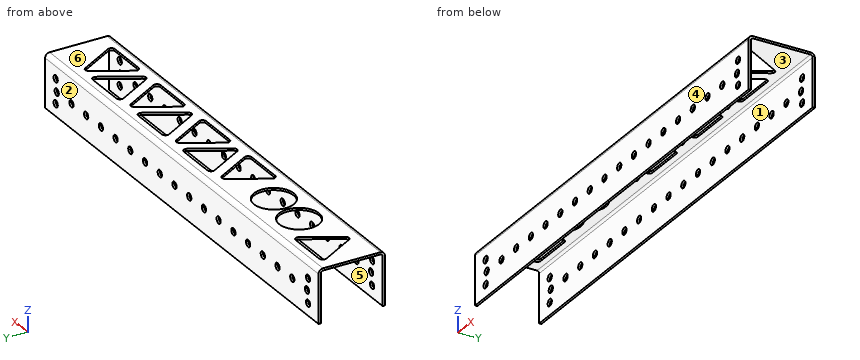
from build123d import *

# Parameters (mm, degrees)
BASE_FLANGE1_DEPTH = 165.1
SKETCH6_R          = 2.54
CUT_EXTRUDE1_DEPTH = 173.973769801
SKETCH8_R          = 14.2875
CUT_EXTRUDE2_DEPTH = 172.104223081
SKETCH9_R          = 14.2875
CUT_EXTRUDE3_DEPTH = 2.54
CUT_EXTRUDE4_DEPTH = 2.54
SKETCH11_R         = 2.54
CUT_EXTRUDE5_DEPTH = 173.973769801


# Sheet-metal steps are written as plain solids
with BuildPart() as part:
    # Sketch1 → Base-Flange1 (new, symmetric)
    with BuildSketch(Plane(origin=(0, 0, 0), x_dir=(0, 0, -1), z_dir=(1, 0, 0))):
        with BuildLine():
            Line((18.25625, 22.225), (-16.66875, 22.225))
            ThreePointArc((-16.66875, 22.225), (-17.791282015, 21.760032015), (-18.25625, 20.6375))
            Line((-18.25625, 20.6375), (-18.25625, -20.6375))
            ThreePointArc((-18.25625, -20.6375), (-17.791282015, -21.760032015), (-16.66875, -22.225))
            Line((-16.66875, -22.225), (18.25625, -22.225))
            Line((18.25625, -22.225), (18.25625, -23.8125))
            Line((18.25625, -23.8125), (-16.66875, -23.8125))
            ThreePointArc((-16.66875, -23.8125), (-18.91381403, -22.88256403), (-19.84375, -20.6375))
            Line((-19.84375, -20.6375), (-19.84375, 20.6375))
            ThreePointArc((-19.84375, 20.6375), (-18.91381403, 22.88256403), (-16.66875, 23.8125))
            Line((-16.66875, 23.8125), (18.25625, 23.8125))
            Line((18.25625, 23.8125), (18.25625, 22.225))
        make_face()
    extrude(amount=BASE_FLANGE1_DEPTH, both=True)

    # Sketch6 → Cut-Extrude1 (cut, through all)
    with BuildSketch(Plane(origin=(0, 23.8125, 0), x_dir=(1, 0, 0), z_dir=(0, 1, 0))):
        with Locations(Location((151.13, 0.79375, 0), (0, 0, 270))):
            Circle(SKETCH6_R)
        with Locations(Location((133.35, 0.79375, 0), (0, 0, 270))):
            Circle(SKETCH6_R)
        with Locations(Location((115.57, 0.79375, 0), (0, 0, 270))):
            Circle(SKETCH6_R)
        with Locations(Location((97.79, 0.79375, 0), (0, 0, 270))):
            Circle(SKETCH6_R)
        with Locations(Location((80.01, 0.79375, 0), (0, 0, 270))):
            Circle(SKETCH6_R)
        with Locations(Location((62.23, 0.79375, 0), (0, 0, 270))):
            Circle(SKETCH6_R)
        with Locations(Location((44.45, 0.79375, 0), (0, 0, 270))):
            Circle(SKETCH6_R)
        with Locations(Location((26.67, 0.79375, 0), (0, 0, 270))):
            Circle(SKETCH6_R)
        with Locations(Location((8.89, 0.79375, 0), (0, 0, 270))):
            Circle(SKETCH6_R)
        with Locations(Location((-8.89, 0.79375, 0), (0, 0, 270))):
            Circle(SKETCH6_R)
        with Locations(Location((-26.67, 0.79375, 0), (0, 0, 270))):
            Circle(SKETCH6_R)
        with Locations(Location((-44.45, 0.79375, 0), (0, 0, 270))):
            Circle(SKETCH6_R)
        with Locations(Location((-62.23, 0.79375, 0), (0, 0, 270))):
            Circle(SKETCH6_R)
        with Locations(Location((-80.01, 0.79375, 0), (0, 0, 270))):
            Circle(SKETCH6_R)
        with Locations(Location((-97.79, 0.79375, 0), (0, 0, 270))):
            Circle(SKETCH6_R)
        with Locations(Location((-115.57, 0.79375, 0), (0, 0, 270))):
            Circle(SKETCH6_R)
        with Locations(Location((-133.35, 0.79375, 0), (0, 0, 270))):
            Circle(SKETCH6_R)
        with Locations(Location((-151.13, 0.79375, 0), (0, 0, 270))):
            Circle(SKETCH6_R)
    extrude(amount=-CUT_EXTRUDE1_DEPTH, mode=Mode.SUBTRACT)

    # Sketch8 → Cut-Extrude2 (cut, through all)
    with BuildSketch(Plane.XY.offset(19.84375)):
        with Locations((-101.6, 0)):
            Circle(SKETCH8_R)
    extrude(amount=-CUT_EXTRUDE2_DEPTH, mode=Mode.SUBTRACT)

    # Sketch9 → Cut-Extrude3 (cut)
    with BuildSketch(Plane.XY.offset(19.84375)):
        with Locations((-71.12, 0)):
            Circle(SKETCH9_R)
        with BuildLine():
            Line((135.902216058, 12.3825), (150.200295474, -12.3825))
            ThreePointArc((150.200295474, -12.3825), (150.200295474, -14.9225), (148.000590949, -16.1925))
            Line((148.000590949, -16.1925), (119.404432116, -16.1925))
            ThreePointArc((119.404432116, -16.1925), (117.20472759, -14.9225), (117.20472759, -12.3825))
            Line((117.20472759, -12.3825), (131.502807007, 12.3825))
            ThreePointArc((131.502807007, 12.3825), (133.702511532, 13.6525), (135.902216058, 12.3825))
        make_face()
        with BuildLine():
            Line((91.908125546, 16.1925), (120.504284379, 16.1925))
            ThreePointArc((120.504284379, 16.1925), (122.703988904, 14.9225), (122.703988904, 12.3825))
            Line((122.703988904, 12.3825), (108.405909488, -12.3825))
            ThreePointArc((108.405909488, -12.3825), (106.206204962, -13.6525), (104.006500437, -12.3825))
            Line((104.006500437, -12.3825), (89.70842102, 12.3825))
            ThreePointArc((89.70842102, 12.3825), (89.70842102, 14.9225), (91.908125546, 16.1925))
        make_face()
        with BuildLine():
            Line((62.21211445, -12.3825), (76.510193866, 12.3825))
            ThreePointArc((76.510193866, 12.3825), (78.709898392, 13.6525), (80.909602918, 12.3825))
            Line((80.909602918, 12.3825), (95.207682334, -12.3825))
            ThreePointArc((95.207682334, -12.3825), (95.207682334, -14.9225), (93.007977808, -16.1925))
            Line((93.007977808, -16.1925), (64.411818976, -16.1925))
            ThreePointArc((64.411818976, -16.1925), (62.21211445, -14.9225), (62.21211445, -12.3825))
        make_face()
        with BuildLine():
            Line((34.71580788, 12.3825), (49.013887296, -12.3825))
            ThreePointArc((49.013887296, -12.3825), (51.213591822, -13.6525), (53.413296347, -12.3825))
            Line((53.413296347, -12.3825), (67.711375764, 12.3825))
            ThreePointArc((67.711375764, 12.3825), (67.711375764, 14.9225), (65.511671238, 16.1925))
            Line((65.511671238, 16.1925), (36.915512405, 16.1925))
            ThreePointArc((36.915512405, 16.1925), (34.71580788, 14.9225), (34.71580788, 12.3825))
        make_face()
        with BuildLine():
            Line((21.517580726, 12.3825), (7.21950131, -12.3825))
            ThreePointArc((7.21950131, -12.3825), (7.21950131, -14.9225), (9.419205835, -16.1925))
            Line((9.419205835, -16.1925), (38.015364668, -16.1925))
            ThreePointArc((38.015364668, -16.1925), (40.215069194, -14.9225), (40.215069194, -12.3825))
            Line((40.215069194, -12.3825), (25.916989777, 12.3825))
            ThreePointArc((25.916989777, 12.3825), (23.717285252, 13.6525), (21.517580726, 12.3825))
        make_face()
        with BuildLine():
            Line((-18.077100735, 16.1925), (10.519058098, 16.1925))
            ThreePointArc((10.519058098, 16.1925), (12.718762624, 14.9225), (12.718762624, 12.3825))
            Line((12.718762624, 12.3825), (-1.579316793, -12.3825))
            ThreePointArc((-1.579316793, -12.3825), (-3.779021318, -13.6525), (-5.978725844, -12.3825))
            Line((-5.978725844, -12.3825), (-20.276805261, 12.3825))
            ThreePointArc((-20.276805261, 12.3825), (-20.276805261, 14.9225), (-18.077100735, 16.1925))
        make_face()
        with BuildLine():
            Line((-33.475032414, 12.3825), (-47.773111831, -12.3825))
            ThreePointArc((-47.773111831, -12.3825), (-47.773111831, -14.9225), (-45.573407305, -16.1925))
            Line((-45.573407305, -16.1925), (-16.977248472, -16.1925))
            ThreePointArc((-16.977248472, -16.1925), (-14.777543947, -14.9225), (-14.777543947, -12.3825))
            Line((-14.777543947, -12.3825), (-29.075623363, 12.3825))
            ThreePointArc((-29.075623363, 12.3825), (-31.275327889, 13.6525), (-33.475032414, 12.3825))
        make_face()
    extrude(amount=-CUT_EXTRUDE3_DEPTH, mode=Mode.SUBTRACT)

    # Sketch10 → Cut-Extrude4 (cut)
    with BuildSketch(Plane.XY.offset(19.84375)):
        with BuildLine():
            Line((-155.280295474, 12.3825), (-140.982216058, -12.3825))
            ThreePointArc((-140.982216058, -12.3825), (-138.782511532, -13.6525), (-136.582807007, -12.3825))
            Line((-136.582807007, -12.3825), (-122.28472759, 12.3825))
            ThreePointArc((-122.28472759, 12.3825), (-122.28472759, 14.9225), (-124.484432116, 16.1925))
            Line((-124.484432116, 16.1925), (-153.080590949, 16.1925))
            ThreePointArc((-153.080590949, 16.1925), (-155.280295474, 14.9225), (-155.280295474, 12.3825))
        make_face()
    extrude(amount=-CUT_EXTRUDE4_DEPTH, mode=Mode.SUBTRACT)

    # Sketch11 → Cut-Extrude5 (cut, through all)
    with BuildSketch(Plane(origin=(0, 23.8125, 0), x_dir=(1, 0, 0), z_dir=(0, 1, 0))):
        with Locations(Location((152.4, 9.525, 0), (0, 0, 270))):
            Circle(SKETCH11_R)
        with Locations(Location((152.4, -7.9375, 0), (0, 0, 270))):
            Circle(SKETCH11_R)
        with Locations(Location((-152.4, -7.9375, 0), (0, 0, 270))):
            Circle(SKETCH11_R)
        with Locations(Location((-152.4, 9.525, 0), (0, 0, 270))):
            Circle(SKETCH11_R)
    extrude(amount=-CUT_EXTRUDE5_DEPTH, mode=Mode.SUBTRACT)


solid = part.part
Read the model definition and answer for the solid it produces. Units are mm, in the model's axes. Face numbers are marked on the shaded views. A direction names the side the tool comes from. Coordinates: 2 decimals unless noted, no trailing zeros. Put each result on its own line as item: value. Start each with the question number.
Item 1: Given pin 1 Ø3 at (x, z) = (-152.4, 7.94) entering from +Y; pin 2 Ø8 at (x, z) = (44.45, -0.79) entering from +Y; pin 3 Ø10 at (x, y) = (117, -5.5) entering from -Z, each flat-ended and moving along its own axis, determine where each tip first touches the part or whether it passes through.
Item 2: Consider probe 1 along Y at (x, z) = (56, -6) (1 decimal); probe 2 along Z at (x, y) = (-46.5, 14); probe 3 along Z at (x, y) = (-133.35, -22.7). Determine where each line is inside the solid, lowest interval first. Write a range as [from, to].
Item 3: Section A-A, the plane y = -8 is taken. Count the separate pieces of the cut face and the enclosed holes in it, plus the area to 3 significant figures.
Item 4: The mould has two halves that part along Y. Classify the marked faces 3, 4, 5 and 6: +Y half, -Y half, draft (parallel to the pull), parting line (faces both ways), or undercut.
Item 5: For the marked faces 1 and 2, determine the directions among +Z, -Z, +X, -X, +Y, -Y from which every point of the face is accessible in a straight line to the end or side of a thin tool.
Computed:
1. pin 1: passes through
1. pin 2: stops at y = 23.81
1. pin 3: stops at z = 18.26
2. probe 1: y = [-23.8, -22.2], [22.2, 23.8]
2. probe 2: z = [18.26, 19.84]
2. probe 3: z = [-18.26, -3.33], [1.75, 19.08]
3. separate pieces: 11
3. enclosed holes: 0
3. area: 212 mm2
4. face 3: undercut
4. face 4: -Y half
4. face 5: undercut
4. face 6: draft
5. face 1: -Z, +X, -X
5. face 2: +Z, -Z, +X, -X, +Y
